from build123d import *

# Parameters (mm, degrees)
SKETCH3_R      = 0.97155
EXTRUDE2_DEPTH = 2.41
CHAMFER1_SIZE  = 0.25


with BuildPart() as part:
    # Sketch2 → Revolve1 (revolve)
    with BuildSketch(Plane(origin=(0, 0, 0), x_dir=(0, 0, -1), z_dir=(1, 0, 0))):
        with BuildLine():
            Line((-7.62, 0), (-11.5062, 0))
            Line((-11.5062, 0), (-11.5062, 8.178792884))
            ThreePointArc((-11.5062, 8.178792884), (-11.134225612, 9.076818496), (-10.2362, 9.448792884))
            Line((-10.2362, 9.448792884), (-8.483598247, 9.448792884))
            ThreePointArc((-8.483598247, 9.448792884), (-8.303993125, 9.523187762), (-8.229598247, 9.702792884))
            Line((-8.229598247, 9.702792884), (-8.229598247, 10.566392884))
            ThreePointArc((-8.229598247, 10.566392884), (-8.15520337, 10.745998007), (-7.975598247, 10.820392884))
            Line((-7.975598247, 10.820392884), (-2.895598247, 10.820392884))
            Line((-2.895598247, 10.820392884), (-2.895598247, 10.464792884))
            Line((-2.895598247, 10.464792884), (0, 10.464792884))
            Line((0, 10.464792884), (0, 5.08))
            Line((0, 5.08), (-7.62, 5.08))
            Line((-7.62, 5.08), (-7.62, 0))
        make_face()
    revolve(axis=Axis((0, 0, 0), (0, 0, 1)))

    # Sketch3 → Extrude2 (add)
    with BuildSketch(Plane.XY):
        with Locations((7.4422, 0)):
            Circle(SKETCH3_R)
        with Locations(Location((-7.4422, 0, 0), (0, 0, 90))):
            Circle(SKETCH3_R)
    extrude(amount=-EXTRUDE2_DEPTH)

    # Chamfer1
    chamfer1_edges = [part.edges().sort_by_distance(p)[0] for p in [
        (6.47065, 0, -2.41),
        (-7.4422, -0.97155, -2.41),
    ]]
    chamfer(chamfer1_edges, length=CHAMFER1_SIZE)


solid = part.part
Geometry: final body of the model. Coordinates: model frame, mm. A direction names the side the tool comes from. Give positions to 0.01 mm unless a question says otherwise; leave off trailing zeros. Order: outer loops, then holes, each group sorted by start corner. A loop starts at its lowest first (then second) coordinate and runs counter-clockwise, first axis right, second up. Notation, with made-up numbers: (68.5, 22) - (113.5, 22) arc R16 cw to (113.5, 35) - close; hole circle Ø11 at (48.5, 0). An arc over 180 degrees is marked (long way). Use CSV: the item, a comma, the result in double quotes.
1. Contact query for flat-ended pins moving along their axis: pin 1 (2 mm diameter, centred on x = 0.5, y = 5.5, fed in from -Z); pin 2 (3 mm diameter, centred on y = 6, z = 6.5, fed in from +X); pin 3 (5 mm diameter, centred on x = -2, y = -1.5, fed in from -Z). Output: stop coordinate, or through.
Answers below:
pin 1,"z = 0"
pin 2,"x = 9.84"
pin 3,"z = 7.62"
2. Section query A-A (x = 0). Output: boundary loops of the cut face in (y, z), plus the area to 3 significant figures.
Answers below:
outline,"(-10.82, 2.9) - (-10.46, 2.9) - (-10.46, 0) - (-5.08, 0) - (-5.08, 7.62) - (5.08, 7.62) - (5.08, 0) - (10.46, 0) - (10.46, 2.9) - (10.82, 2.9) - (10.82, 7.98) arc R0.25 ccw to (10.57, 8.23) - (9.7, 8.23) arc R0.25 cw to (9.45, 8.48) - (9.45, 10.24) arc R1.27 ccw to (8.18, 11.51) - (-8.18, 11.51) arc R1.27 ccw to (-9.45, 10.24) - (-9.45, 8.48) arc R0.25 cw to (-9.7, 8.23) - (-10.57, 8.23) arc R0.25 ccw to (-10.82, 7.98) - close"
area,"160 mm2"
3. Section query C-C (z = 5.5). Output: boundary loops of the cut face in (x, y).
Answers below:
outline,"circle Ø21.64 at (0, 0); hole circle Ø10.16 at (0, 0)"
4. Material intervals for line 1 along X through (y, z) = (0, 2.75); line 2 along X through (y, z) = (0, 3), sorted ascending. Write a range as from..to.
Answers below:
line 1,"-10.46..-5.08, 5.08..10.46"
line 2,"-10.82..-5.08, 5.08..10.82"
5. Mould query, pull axis Y, two halves, no side actions, for faces 4 (the face through (-5.037, -0.661, 3.863)), 5 (the face through (7, 0, -2.41)), 6 (the face through (-8.405, -0.126, -1.065)). Classes: +Y half, -Y half, draft (parallel to the pull), parting line (faces both ways), or undercut.
Answers below:
face 4,"undercut"
face 5,"draft"
face 6,"parting line"
6. Access query for faces 1 (the face through (10.563, -2.346, 5.4)), 2 (the face through (0, 0, 7.62)), 3 (the face through (5, -9, 8.23)). Directions: +Z, -Z, +X, -X, +Y, -Y. A direction counts if a zero-diameter tool reaches every point of the face in a straight line with its end or side. Return the directions, or none.
Answers below:
face 1,"+Z, -Z"
face 2,"-Z"
face 3,"+Z"
